```python
from build123d import *

# Parameters (mm, degrees)
F0_W        = 78.6384046078
F0_H        = 133.1976056099
F0_W_2      = 69.4944038987
F0_H_2      = 123.444005847
F1_DEPTH    = 12.7
F2_T1_DEPTH = 83.6549732601
F2_T3_DEPTH = 136.8933778678


# Not quite as in the source:
# - a fillet or chamfer that OpenCascade refuses, or shapes differently, is made with other operations: its cross-section is extruded or revolved along the edge and cut away or added


with BuildPart() as f1:
    # F0 (on Front) → F1 (new body, symmetric)
    with BuildSketch(Plane.XZ):
        Rectangle(F0_W, F0_H)
        Rectangle(F0_W_2, F0_H_2, mode=Mode.SUBTRACT)
    extrude(amount=F1_DEPTH, both=True)

    # F2: fillet of radius 11.650994652 on 8 edges, made by hand

    # F2_s2 → F2_t1 (cut)
    with BuildSketch(Plane.XZ.offset(-41.82748663)):
        with BuildLine():
            ThreePointArc((39.3192023039, 54.9478081529), (35.9067049779, 63.1863054789), (27.6682076519, 66.5988028049))
            Line((27.6682076519, 66.5988028049), (39.3192023039, 66.5988028049))
            Line((39.3192023039, 66.5988028049), (39.3192023039, 54.9478081529))
        make_face()
        with BuildLine():
            ThreePointArc((-39.3192023039, 54.9478081529), (-35.9067049779, 63.1863054789), (-27.6682076519, 66.5988028049))
            Line((-27.6682076519, 66.5988028049), (-39.3192023039, 66.5988028049))
            Line((-39.3192023039, 66.5988028049), (-39.3192023039, 54.9478081529))
        make_face()
        with BuildLine():
            ThreePointArc((39.3192023039, -54.9478081529), (35.9067049779, -63.1863054789), (27.6682076519, -66.5988028049))
            Line((27.6682076519, -66.5988028049), (39.3192023039, -66.5988028049))
            Line((39.3192023039, -66.5988028049), (39.3192023039, -54.9478081529))
        make_face()
        with BuildLine():
            ThreePointArc((-27.6682076519, -66.5988028049), (-35.9067049779, -63.1863054789), (-39.3192023039, -54.9478081529))
            Line((-39.3192023039, -54.9478081529), (-39.3192023039, -66.5988028049))
            Line((-39.3192023039, -66.5988028049), (-27.6682076519, -66.5988028049))
        make_face()
    extrude(amount=F2_T1_DEPTH, mode=Mode.SUBTRACT)

    # F2_s4 → F2_t3 (cut)
    with BuildSketch(Plane.YZ.offset(-68.4466889339)):
        with BuildLine():
            ThreePointArc((1.049005348, 66.5988028049), (9.287502674, 63.1863054789), (12.7, 54.9478081529))
            Line((12.7, 54.9478081529), (12.7, 66.5988028049))
            Line((12.7, 66.5988028049), (1.049005348, 66.5988028049))
        make_face()
        with BuildLine():
            ThreePointArc((-12.7, 54.9478081529), (-9.287502674, 63.1863054789), (-1.049005348, 66.5988028049))
            Line((-1.049005348, 66.5988028049), (-12.7, 66.5988028049))
            Line((-12.7, 66.5988028049), (-12.7, 54.9478081529))
        make_face()
        with BuildLine():
            ThreePointArc((1.049005348, -66.5988028049), (9.287502674, -63.1863054789), (12.7, -54.9478081529))
            Line((12.7, -54.9478081529), (12.7, -66.5988028049))
            Line((12.7, -66.5988028049), (1.049005348, -66.5988028049))
        make_face()
        with BuildLine():
            ThreePointArc((-1.049005348, -66.5988028049), (-9.287502674, -63.1863054789), (-12.7, -54.9478081529))
            Line((-12.7, -54.9478081529), (-12.7, -66.5988028049))
            Line((-12.7, -66.5988028049), (-1.049005348, -66.5988028049))
        make_face()
    extrude(amount=F2_T3_DEPTH, mode=Mode.SUBTRACT)


solid = f1.part
```
Read the model definition and answer for the solid it produces. Units are mm, in the model's axes. A direction names the side the tool comes from. Coordinates: 2 decimals unless noted, no trailing zeros. Write each loop counter-clockwise with the first axis right and the second up, starting at its lowest first coordinate (ties: lowest second). Pieces come first, ordered by that corner, then holes. Notation, with made-up numbers: (86.25, -33.5) -> (140.25, -33.5) arc R12 cw to (140.25, -18.5) -> close; hole circle Ø5 at (3.5, -1.75). An arc over 180 degrees is marked (long way). Answer as a JSON object with one key per item and string values.
Q1. A tool of negligible diameter and unlimited length cuts with its end or side. For faces 4 (the flat face through (0, 0, -61.722)), 5 (the cylindrical face through (-0.55, 7.63, 64.56)), from which of +Z, -Z, +X, -X, +Y, -Y can it reach the whole face along a straight path? Write none if from no direction.
The answers:
{"face 4": "+Y, -Y", "face 5": "+Z, +X, -X, +Y"}
Q2. The part is cut by section B-B on x = 3.5. Give the vertices of the cut face in (y, z).
The answers:
{"outline": "(-10.53, -61.72) arc R11.65 ccw to (-1.05, -66.6) -> (1.05, -66.6) arc R11.65 ccw to (10.53, -61.72) -> close; (-10.53, 61.72) -> (10.53, 61.72) arc R11.65 ccw to (1.05, 66.6) -> (-1.05, 66.6) arc R11.65 ccw to start"}
Q3. The part is cut by section A-A on z = -11.5. Give the vertices of the cut face in (x, y).
The answers:
{"outline": "(-39.32, -12.7) -> (-34.75, -12.7) -> (-34.75, 12.7) -> (-39.32, 12.7) -> close; (34.75, -12.7) -> (39.32, -12.7) -> (39.32, 12.7) -> (34.75, 12.7) -> close"}
Q4. The part is cut by section D-D on y = 9. Give the vertices of the cut face in (x, z), then the cut area to 3 significant figures.
The answers:
{"outline": "(-39.32, -54.95) arc R11.65 ccw to (-35.62, -63.46) -> (35.62, -63.46) arc R11.65 ccw to (39.32, -54.95) -> (39.32, 54.95) arc R11.65 ccw to (35.62, 63.46) -> (-35.62, 63.46) arc R11.65 ccw to (-39.32, 54.95) -> close; hole (-34.75, -61.72) -> (34.75, -61.72) -> (34.75, 61.72) -> (-34.75, 61.72) -> close", "area": "1,360 mm2"}
Q5. Consider line 1 (X direction, y = -1, z = -49); line 2 (Z direction, x = -25.5, y = -0.75); line 3 (Z direction, x = 17, y = -9.25). Determine where each line is inside the solid, lowest interval first. Write a range as [from, to].
The answers:
{"line 1": "x = [-39.32, -34.75], [34.75, 39.32]", "line 2": "z = [-66.6, -61.72], [61.72, 66.6]", "line 3": "z = [-63.22, -61.72], [61.72, 63.22]"}
Q6. The part is cut by section C-C on y = -6.25. Give the vertices of the cut face in (x, z).
The answers:
{"outline": "(-39.32, -54.95) arc R11.65 ccw to (-32.87, -65.37) -> (32.87, -65.37) arc R11.65 ccw to (39.32, -54.95) -> (39.32, 54.95) arc R11.65 ccw to (32.87, 65.37) -> (-32.87, 65.37) arc R11.65 ccw to (-39.32, 54.95) -> close; hole (-34.75, -61.72) -> (34.75, -61.72) -> (34.75, 61.72) -> (-34.75, 61.72) -> close"}
Q7. Flat-ended cylindrical pins translate along their axes: pin 1 Ø1.5 at (x, y) = (7, 7.5) entering from +Z; pin 2 Ø1.5 at (x, y) = (-25, 2.5) entering from +Z. Find the tip coordinate at first contact, or state that the pin passes through.
The answers:
{"pin 1": "stops at z = 65.11", "pin 2": "stops at z = 66.58"}
Q8. Determine the mould class of faces 1 (the flat face through (-37, 12.7, 1)), 2 (the flat face through (0, 0, 61.722)), 3 (the cylindrical face through (37.3, 0.2, -61.5)) for opening direction X: pulls with the +X half, pulls with the -X half, needs draft (parallel to the pull), parting line crosses it, or undercut.
The answers:
{"face 1": "needs draft", "face 2": "undercut", "face 3": "pulls with the +X half"}
